Verification items for this drawing (mm, ordinates from the low corner). A direction names the side the tool comes from. Coordinates: 2 decimals unless noted, no trailing zeros. Order: outer loops, then holes, each group sorted by start corner. A loop starts at its lowest first (then second) coordinate and runs counter-clockwise, first axis right, second up.
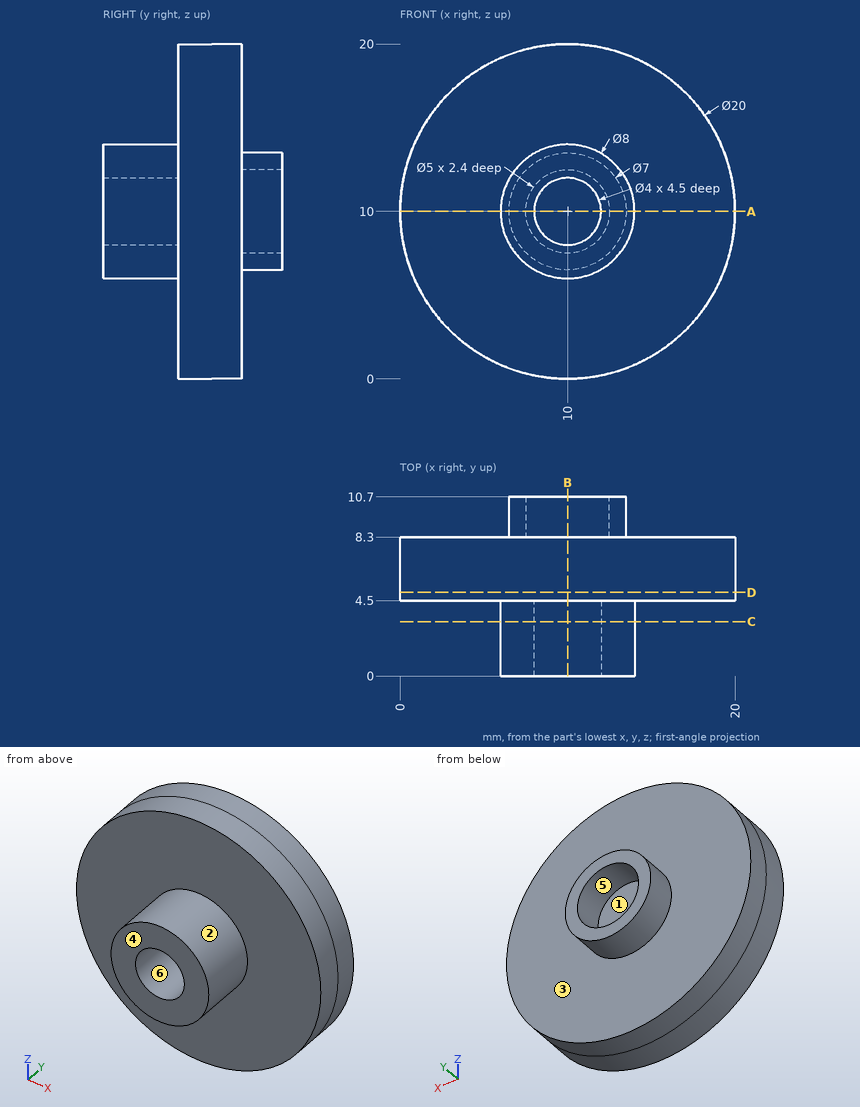
Item 1: Depth check by flat-ended pin: P1, Ø4.5, axis at x = 10, z = 10, coming from the +Y side; P2, Ø12, axis at x = 2.5, z = 15, coming from the -Y side; P3, Ø1.5, axis at x = 14, y = 8, coming from the +Z side; P4, Ø2, axis at y = 6, z = 7.5, coming from the +X side. Enter the tip coordinate at first touch or a pass-through.
Item 2: Sectioned sample at C-C (y = 3.25). Record the cut outline in (x, z).
Item 3: Thickness scan on line 1 along X through (y, z) = (9.6, 10); line 2 along Z through (x, y) = (10, 2.25). Record the ranges inside material, lowest first.
Item 4: Sectioned sample at D-D (y = 5). Record the cut outline in (x, z).
Item 5: Tool access check on the marked faces 4, 5 and 6. Record the directions out of +Z, -Z, +X, -X, +Y, -Y that give a thin tool (end or side, any length) a straight path to the whole face; none if there is none.
Item 6: Release check for a two-part mould opening along X. For the marked faces 1, 2 and 3 record: pulls with the +X half, pulls with the -X half, needs draft (parallel to the pull), parting line crosses it, or undercut.
Item 7: Sectioned sample at B-B (x = 10). Record the cut outline in (y, z).
Item 8: Sectioned sample at A-A (z = 10). Record the cut outline in (x, y).
Geometry check:
1. P1: stops at y = 8.3
1. P2: stops at y = 0
1. P3: stops at z = 19.46
1. P4: stops at x = 19.89
2. outline: circle Ø8 at (10, 10); hole circle Ø4 at (10, 10)
3. line 1: x = 6.5 to 7.5, 12.5 to 13.5
3. line 2: z = 6 to 8, 12 to 14
4. outline: circle Ø20 at (10, 10)
5. face 4: +Z, -Z, +X, -X, -Y
5. face 5: +Y
5. face 6: -Y
6. face 1: undercut
6. face 2: parting line crosses it
6. face 3: needs draft
7. outline: (0, 6) - (4.5, 6) - (4.5, 0) - (8.3, 0) - (8.3, 6.5) - (10.7, 6.5) - (10.7, 7.5) - (8.3, 7.5) - (8.3, 12.5) - (10.7, 12.5) - (10.7, 13.5) - (8.3, 13.5) - (8.3, 20) - (4.5, 20) - (4.5, 14) - (0, 14) - (0, 12) - (4.5, 12) - (4.5, 8) - (0, 8) - close
8. outline: (0, 4.5) - (6, 4.5) - (6, 0) - (8, 0) - (8, 4.5) - (12, 4.5) - (12, 0) - (14, 0) - (14, 4.5) - (20, 4.5) - (20, 8.3) - (13.5, 8.3) - (13.5, 10.7) - (12.5, 10.7) - (12.5, 8.3) - (7.5, 8.3) - (7.5, 10.7) - (6.5, 10.7) - (6.5, 8.3) - (0, 8.3) - close
